Geometry check sheet. Reference: the model listing, model coordinates, mm. A direction names the side the tool comes from. Give positions to 0.01 mm unless a question says otherwise; leave off trailing zeros. Loops run counter-clockwise (first coordinate to the right, second up) from the corner with the lowest first, then second, coordinate; pieces in that order, holes last. Notation, with made-up numbers: (87.5, 36) -> (144.5, 36) arc R29 cw to (144.5, 57) -> close; hole circle Ø2 at (-37.5, 52). An arc over 180 degrees is marked (long way). One line per item, written item: value. Start each with the question number.
(1) Draft check along Z on faces 1 (the face through (-6, -9.369, 13)), 2 (the face through (0, -22, 2.54)), 3 (the face through (-6, -22, 25.4)). Enter one of: pulls with the +Z half, pulls with the -Z half, needs draft (parallel to the pull), parting line crosses it, or undercut.
(2) Sectioned sample at A-A, the plane x = -120. Record the cut outline in (y, z), then the cut area to 3 significant figures.
(3) Tool access check on faces 4 (the face through (-6, -34.769, 13)), 5 (the face through (0, -32.229, 8)). Record the directions out of +Z, -Z, +X, -X, +Y, -Y that give a thin tool (end or side, any length) a straight path to the whole face; none if there is none.
(4) Scan lines: line 1 along Y through (x, z) = (-154.5, 13.25); line 2 along Z through (x, y) = (115, -24.5); line 3 along Z through (x, y) = (-128, -11). Record each from-to range of solid material in increasing order. Write a range as from..to.
from build123d import *

# Parameters (mm, degrees)
F0_W     = 431.8
F0_H     = 25.4
F1_DEPTH = 25.4
F2_W     = 20.32
F2_H     = 20.32
F3_DEPTH = 457.2
F5_D     = 5.1054
F7_D     = 5.1054


with BuildPart() as f1:
    # F0 (on Top) → F1 (new body)
    with BuildSketch(Plane.XY):
        with Locations((-2.601906, -22.068714)):
            Rectangle(F0_W, F0_H)
    extrude(amount=F1_DEPTH)

    # F2 (on face) → F3 (cut)
    with BuildSketch(Plane.YZ.offset(213.298094)):
        with Locations((-22.068714, 12.7)):
            Rectangle(F2_W, F2_H)
    extrude(amount=-F3_DEPTH, mode=Mode.SUBTRACT)

    # F5 (through all)
    with Locations(Plane.XY.offset(25.4)):
        with Locations((200.313424, -22.068714), (149.513424, -22.068714), (225.713424, -22.068714), (73.313424, -22.068714), (98.713424, -22.068714), (124.113424, -22.068714), (-206.086576, -22.068714), (-180.686576, -22.068714), (-155.286576, -22.068714), (-129.886576, -22.068714), (-104.486576, -22.068714), (-79.086576, -22.068714), (-53.686576, -22.068714), (174.913424, -22.068714), (-28.286576, -22.068714), (-2.886576, -22.068714), (22.513424, -22.068714), (47.913424, -22.068714)):
            Hole(F5_D / 2)

    # F7 (through all)
    with Locations(Plane(origin=(0, -9.368714, 0), x_dir=(-1, 0, 0), z_dir=(0, 1, 0))):
        with Locations((177.082395, 12.7), (151.682395, 12.7), (-229.317605, 12.7), (-178.517605, 12.7), (-203.917605, 12.7), (-127.717605, 12.7), (-153.117605, 12.7), (50.082395, 12.7), (100.882395, 12.7), (75.482395, 12.7), (202.482395, 12.7), (126.282395, 12.7), (-76.917605, 12.7), (-102.317605, 12.7), (-26.117605, 12.7), (-51.517605, 12.7), (24.682395, 12.7), (-0.717605, 12.7)):
            Hole(F7_D / 2)


solid = f1.part
Calculated:
1. face 1: needs draft
1. face 2: undercut
1. face 3: pulls with the +Z half
2. outline: (-34.77, 0) -> (-9.37, 0) -> (-9.37, 25.4) -> (-34.77, 25.4) -> close; hole (-32.23, 2.54) -> (-11.91, 2.54) -> (-11.91, 22.86) -> (-32.23, 22.86) -> close
2. area: 232 mm2
3. face 4: +Z, -Z, +X, -X, -Y
3. face 5: +X, -X
4. line 1: y = -34.77..-32.23, -11.91..-9.37
4. line 2: z = 0..2.54, 22.86..25.4
4. line 3: z = 0..10.81, 14.59..25.4
